Read the model definition and answer for the solid it produces. Units are mm, in the model's axes. Face numbers are marked on the shaded views. Coordinates: 2 decimals unless noted, no trailing zeros. Write each loop counter-clockwise with the first axis right and the second up, starting at its lowest first coordinate (ties: lowest second). Pieces come first, ordered by that corner, then holes. Notation, with made-up numbers: (83.5, 34) -> (107.5, 34) arc R20 ccw to (107.5, 73) -> close; hole circle Ø11 at (60.25, -40). An arc over 180 degrees is marked (long way). Write item = value, one per line. Start each with the question number.
1) Flat-ended cylindrical pins translate along their axes: pin 1 Ø8 at (y, z) = (126.5, -16) entering from +X; pin 2 Ø7 at (x, z) = (0, 60) entering from +Y; pin 3 Ø4 at (y, z) = (193.5, -30) entering from -X. Find the tip coordinate at first contact, or state that the pin passes through.
2) Section A-A (z = 0) is taken. Determine the outline of the cut face in (x, y).
3) Find the intervals of material crossed by line 1 along X through (y, z) = (3.4, 0); line 2 along Y through (x, z) = (69, 15); line 3 along Y through (x, z) = (18.5, 66), in increasing order. Write a range as from..to.
4) Section B-B (x = 0) is taken. Determine the outline of the cut face in (y, z), plus the area to 3 significant figures.
5) For a pull along Y with two mould halves and no side action, classify the marked faces 1 and 2 as released by +Y, released by -Y, zero draft, split by the parting line, or undercut.
6) Section C-C (x = -47) is taken. Determine the outline of the cut face in (y, z).
7) Section D-D (z = -73) is taken. Determine the outline of the cut face in (x, y), plus the area to 3 significant figures.
from build123d import *

# Parameters (mm, degrees)
SKETCH_1_R      = 80
EXTRUDE_1_DEPTH = 5
MM_1_D          = 8
MM_1_DEPTH      = 20
MM_1_TIP        = 2.403442476
SKETCH_4_W      = 15
SKETCH_4_H      = 30


with BuildPart() as part:
    # 草图1 → 凸台-拉伸1 (new body)
    with BuildSketch(Plane(origin=(0, 0, 0), x_dir=(1, 0, 0), z_dir=(0, 1, 0))):
        with Locations(Location((0, 0, 0), (0, 0, 270))):
            Circle(SKETCH_1_R)
    extrude(amount=EXTRUDE_1_DEPTH)

    # 大小mm 暗销孔1
    with Locations(Plane(origin=(0, 5, -60), x_dir=(0, 0, 1), z_dir=(0, 1, 0))):
        with Locations((0, 0), (60, -60), (60, 60), (120, 0)):
            Hole(MM_1_D / 2, depth=MM_1_DEPTH)
            with Locations((0, 0, -(MM_1_DEPTH + MM_1_TIP / 2))):  # 118° drill point
                Cone(0, MM_1_D / 2, MM_1_TIP, mode=Mode.SUBTRACT)

    # 草图4 → 旋转1 (revolve)
    with BuildSketch(Plane.XY, mode=Mode.PRIVATE) as revolve_1_sk:
        with Locations((7.5, 20)):
            Rectangle(SKETCH_4_W, SKETCH_4_H)
    revolve(revolve_1_sk.sketch.rotate(Axis((0, 5, 0), (0, 1, 0)), 90), axis=Axis((0, 5, 0), (0, 1, 0)))

    # 草图5 → 旋转2 (revolve)
    with BuildSketch(Plane.XY):
        with BuildLine():
            Line((0, 35), (0, 30))
            ThreePointArc((0, 30), (-125, 155), (0, 280))
            Line((0, 280), (0, 35))
        make_face()
    revolve(axis=Axis((0, 35, 0), (0, 1, 0)))


solid = part.part
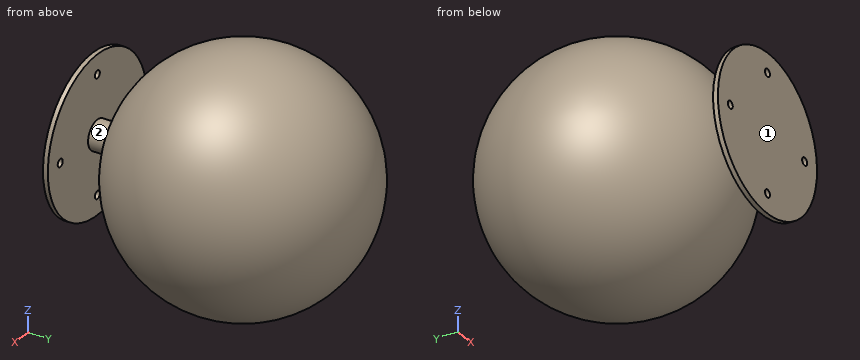
Answer key:
q1.pin_1 = 121.66
q1.pin_2 = 266.5
q1.pin_3 = -115.91
q2.outline = (-80, 0) -> (-64, 0) -> (-64, 5) -> (-80, 5) -> close; (-56, 0) -> (56, 0) -> (56, 5) -> (15, 5) -> (15, 30.9) arc R125 ccw (long way) to (-15, 30.9) -> (-15, 5) -> (-56, 5) -> close; (64, 0) -> (80, 0) -> (80, 5) -> (64, 5) -> close
q3.line_1 = -80..-64, -56..56, 64..80
q3.line_2 = 0..5, 51.85..258.15
q3.line_3 = 0..5, 50.47..259.53
q4.outline = (0, -80) -> (5, -80) -> (5, -64) -> (0, -64) -> close; (0, -56) -> (5, -56) -> (5, -15) -> (30.9, -15) arc R125 ccw (long way) to (30.9, 15) -> (5, 15) -> (5, 56) -> (0, 56) -> close; (0, 64) -> (5, 64) -> (5, 80) -> (0, 80) -> close
q4.area = 50,600 mm^2
q5.face_1 = released by -Y
q5.face_2 = undercut
q6.outline = (0, -64.74) -> (5, -64.74) -> (5, 64.74) -> (0, 64.74) -> close; circle Ø231.65 at (155, 0)
q7.outline = circle Ø202.94 at (0, 155); (-32.73, 0) -> (32.73, 0) -> (32.73, 5) -> (-32.73, 5) -> close
q7.area = 32,700 mm^2
